from build123d import *

# Parameters (mm, degrees)
F0_W     = 118.373677
F0_H     = 116.875283
F1_DEPTH = 12.7
F2_W     = 106.976003
F2_H     = 53.587355
F3_DEPTH = 25.4
F4_W     = 30.09352
F4_H     = 49.528088
F4_W_2   = 47.223489
F4_H_2   = 38.565222
F5_DEPTH = 12.7
F6_W     = 16.616419
F6_H     = 41.588474
F7_DEPTH = 12.7


with BuildPart() as f1:
    # F0 (on Front) → F1 (new body)
    with BuildSketch(Plane.XZ):
        with Locations((136.354491, 2.996803)):
            Rectangle(F0_W, F0_H)
    extrude(amount=F1_DEPTH)

    # F2 (on face) → F3 (join)
    with BuildSketch(Plane(origin=(0, 0, 0), x_dir=(-1, 0, 0), z_dir=(0, 1, 0))):
        with Locations((-131.941452, -26.793677)):
            Rectangle(F2_W, F2_H)
    extrude(amount=F3_DEPTH)

    # F4 (on face) → F5 (join)
    with BuildSketch(Plane(origin=(0, 0, 0), x_dir=(-1, 0, 0), z_dir=(0, 1, 0))):
        with Locations((-179.041378, 29.658426)):
            Rectangle(F4_W, F4_H)
        with Locations((-105.113152, 25.712056)):
            Rectangle(F4_W_2, F4_H_2)
    extrude(amount=F5_DEPTH)

    # F6 (on face) → F7 (join)
    with BuildSketch(Plane(origin=(0, 0, 0), x_dir=(-1, 0, 0), z_dir=(0, 1, 0))):
        with Locations((-90.637371, 21.197991)):
            Rectangle(F6_W, F6_H)
    extrude(amount=F7_DEPTH)


solid = f1.part
Geometry: final body of the model. Coordinates: model frame, mm. A direction names the side the tool comes from. Coordinates: 2 decimals unless noted, no trailing zeros. Order: outer loops, then holes, each group sorted by start corner. A loop starts at its lowest first (then second) coordinate and runs counter-clockwise, first axis right, second up.
(1) Access query for faces 1 (the face through (105, 6, 44.995)), 2 (the face through (78.453, 13, -27)), 3 (the face through (163.995, 6, 29)), 4 (the face through (105, 12.7, 23)). Directions: +Z, -Z, +X, -X, +Y, -Y. A direction counts if a zero-diameter tool reaches every point of the face in a straight line with its end or side. Return the directions, or none.
(2) Material intervals for probe 1 along Z at (x, y) = (101.5, 7); probe 2 along X at (y, z) = (9, 8.5); probe 3 along Y at (x, z) = (88, 24), sorted ascending.
(3) Section query D-D (z = 18). Return the cut outline in (x, y), plus the area to 3 significant figures.
(4) Section query A-A (y = 2). Return the cut outline in (x, z).
(5) First-contact query: pin 1 (4 mm diameter, centred on y = 4.5, z = 23, fed in from -X); pin 2 (4 mm diameter, centred on x = 172.5, y = 7, fed in from +Z); pin 3 (12.5 mm diameter, centred on x = 142, y = 9.5, fed in from -Z); pin 4 (2 mm diameter, centred on y = 14, z = 10, fed in from -X). Flat tips, straight axial feed; report the tip coordinate or a pass-through.
(6) Section query C-C (x = 100.5). Return the cut outline in (y, z).
(7) Section query B-B (z = -35). Return the cut outline in (x, y).
(8) Draft query along X for faces 5 (the face through (179, 6, 54.422)), 6 (the face through (145, 0, 25)), 7 (the face through (195.541, -6, 2)), 8 (the face through (114, 6, 6.429)). Return one class per face: pulls with the +X half, pulls with the -X half, needs draft (parallel to the pull), parting line crosses it, or undercut.
Solution:
1. face 1: +Z, -X, +Y
1. face 2: +Z, -Z, -X, +Y
1. face 3: +Z, +Y
1. face 4: +Z, +X, -X, +Y
2. probe 1: z = -53.59 to 0, 6.43 to 44.99
2. probe 2: x = 81.5 to 128.72, 163.99 to 194.09
2. probe 3: y = -12.7 to 12.7
3. outline: (77.17, -12.7) - (195.54, -12.7) - (195.54, 0) - (194.09, 0) - (194.09, 12.7) - (163.99, 12.7) - (163.99, 0) - (128.72, 0) - (128.72, 12.7) - (81.5, 12.7) - (81.5, 0) - (77.17, 0) - close
3. area: 2,490 mm2
4. outline: (78.45, -53.59) - (185.43, -53.59) - (185.43, 0) - (78.45, 0) - close; (81.5, 6.43) - (82.33, 6.43) - (82.33, 0.4) - (98.95, 0.4) - (98.95, 6.43) - (128.72, 6.43) - (128.72, 44.99) - (81.5, 44.99) - close; (163.99, 4.89) - (194.09, 4.89) - (194.09, 54.42) - (163.99, 54.42) - close
5. pin 1: stops at x = 81.5
5. pin 2: stops at z = 54.42
5. pin 3: stops at z = -53.59
5. pin 4: passes through
6. outline: (-12.7, -55.44) - (0, -55.44) - (0, -53.59) - (25.4, -53.59) - (25.4, 0) - (0, 0) - (0, 6.43) - (12.7, 6.43) - (12.7, 44.99) - (0, 44.99) - (0, 61.43) - (-12.7, 61.43) - close
7. outline: (77.17, -12.7) - (195.54, -12.7) - (195.54, 0) - (185.43, 0) - (185.43, 25.4) - (78.45, 25.4) - (78.45, 0) - (77.17, 0) - close
8. face 5: needs draft
8. face 6: undercut
8. face 7: pulls with the +X half
8. face 8: undercut
